from build123d import *

# Parameters (mm, degrees)
SKETCH_1_W          = 504.54
SKETCH_1_H          = 140
EXTRUDE_1_DEPTH     = 80
SKETCH_2_W          = 464.54
SKETCH_2_H          = 100
CUT_EXTRUDE_1_DEPTH = 60
CUT_EXTRUDE_2_DEPTH = 516.616729364
SKETCH_8_W          = 462.27
SKETCH_8_H          = 18.765324385
CUT_EXTRUDE_3_DEPTH = 15
SKETCH_12_R         = 20
SKETCH_12_R_2       = 10
EXTRUDE_2_DEPTH     = 10


with BuildPart() as part:
    # 草圖1 → 填料-伸長1 (new body)
    with BuildSketch(Plane(origin=(0, 0, 0), x_dir=(1, 0, 0), z_dir=(0, 1, 0))):
        Rectangle(SKETCH_1_W, SKETCH_1_H)
    extrude(amount=EXTRUDE_1_DEPTH)

    # 草圖2 → 除料-伸長1 (cut)
    with BuildSketch(Plane.XZ):
        Rectangle(SKETCH_2_W, SKETCH_2_H)
    extrude(amount=-CUT_EXTRUDE_1_DEPTH, mode=Mode.SUBTRACT)

    # 草圖7 → 除料-伸長2 (cut, through all)
    with BuildSketch(Plane(origin=(252.27, 0, 0), x_dir=(0, 0, -1), z_dir=(1, 0, 0))):
        Polygon((-70, 21.729405289), (31.457073642, 80), (-70, 80), align=None)
    extrude(amount=-CUT_EXTRUDE_2_DEPTH, mode=Mode.SUBTRACT)

    # 草圖8 → 除料-伸長3 (cut)
    with BuildSketch(Plane(origin=(0, 46.570964705, 26.747448081), x_dir=(1, 0, 0), z_dir=(0, 0.8671544755717103, 0.4980392710378893))):
        with Locations((-1.135, 36.346470221)):
            Rectangle(SKETCH_8_W, SKETCH_8_H)
    extrude(amount=-CUT_EXTRUDE_3_DEPTH, mode=Mode.SUBTRACT)

    # 草圖12 → 伸長-薄件2 (add)
    with BuildSketch(Plane.XZ):
        with Locations((37.16174113, 80)):
            Circle(SKETCH_12_R)
        with Locations((37.16174113, 80)):
            Circle(SKETCH_12_R_2, mode=Mode.SUBTRACT)
    extrude(amount=-EXTRUDE_2_DEPTH)


solid = part.part
The model under review builds one solid part; all positions refer to its coordinate system, in mm. A direction names the side the tool comes from. Coordinates: 2 decimals unless noted, no trailing zeros. Loops run counter-clockwise (first coordinate to the right, second up) from the corner with the lowest first, then second, coordinate; pieces in that order, holes last. Notation, with made-up numbers: M 60,13 L 68,13 A19 cw 68,25 Z; hole C -37,66 d11. An arc over 180 degrees is marked long. Put each result on its own line as item: value. Start each with the question number.
Q1. Add section D-D (z = -44.5). Write out the cut boundary in (x, y).
Q2. Clearance check with flat-ended pins moving along their axes: pin 1 (15 mm diameter, centred on x = 33.5, z = 85, fed in from +Y); pin 2 (24 mm diameter, centred on x = 117, y = 16, fed in from +Z). State where each tip first meets the part, or that it passes through.
Q3. Add section B-B (z = 80). Write out the cut boundary in (x, y).
Q4. The part is to be moulded in two halves that separate along X. For faces 4 (the flat face through (-3, 16, 50)), 5 (the flat face through (252.27, 31, -15)), 6 (the flat face through (-4, 39, -70)), say which applies: +X half, -X half, draft (parallel to the pull), parting line (faces both ways), or undercut.
Q5. Add section A-A (x = 84). Write out the cut boundary in (y, z).
Q6. Add section C-C (y = 15.5). Write out the cut boundary in (x, z), and give its area (3 significant figures).
Q7. Wall thickness on line 1 (X direction, y = 12.5, z = 2); line 2 (X direction, y = 7, z = 80); line 3 (Z direction, x = -88, y = 4): over which ranges is each line inside the solid? List them lowest first.
Q8. For faces 1 (the flat face through (-232.27, 26, -1)), 2 (the flat face through (37, 10, 92)), 3 (the flat face through (230, 64, -10)), list the 3-axis set-ups (+Z, -Z, +X, -X, +Y, -Y) from which the entire face can be reached by the end or side of a thin tool; tool diameter is ignored.
Answers:
1. outline: M -252.27,0 L -232.27,0 L -232.27,60 L 232.27,60 L 232.27,0 L 252.27,0 L 252.27,80 L -252.27,80 Z
2. pin 1: stops at y = 10
2. pin 2: stops at z = 70
3. outline: M 17.16,0 L 27.16,0 L 27.16,10 L 17.16,10 Z; M 47.16,0 L 57.16,0 L 57.16,10 L 47.16,10 Z
4. face 4: undercut
4. face 5: +X half
4. face 6: draft
5. outline: M 0,-70 L 80,-70 L 80,-31.46 L 69.35,-12.91 L 60,-18.27 L 60,-50 L 0,-50 Z; M 0,50 L 33.22,50 L 21.73,70 L 0,70 Z
6. outline: M -252.27,-70 L 252.27,-70 L 252.27,70 L -252.27,70 Z; hole M -232.27,-50 L 232.27,-50 L 232.27,50 L -232.27,50 Z
6. area: 24,200 mm^2
7. line 1: x = -252.27 to -232.27, 232.27 to 252.27
7. line 2: x = 17.16 to 27.16, 47.16 to 57.16
7. line 3: z = -70 to -50, 50 to 70
8. face 1: -Y
8. face 2: +Z, +X, -X, +Y
8. face 3: +Z, -Y
